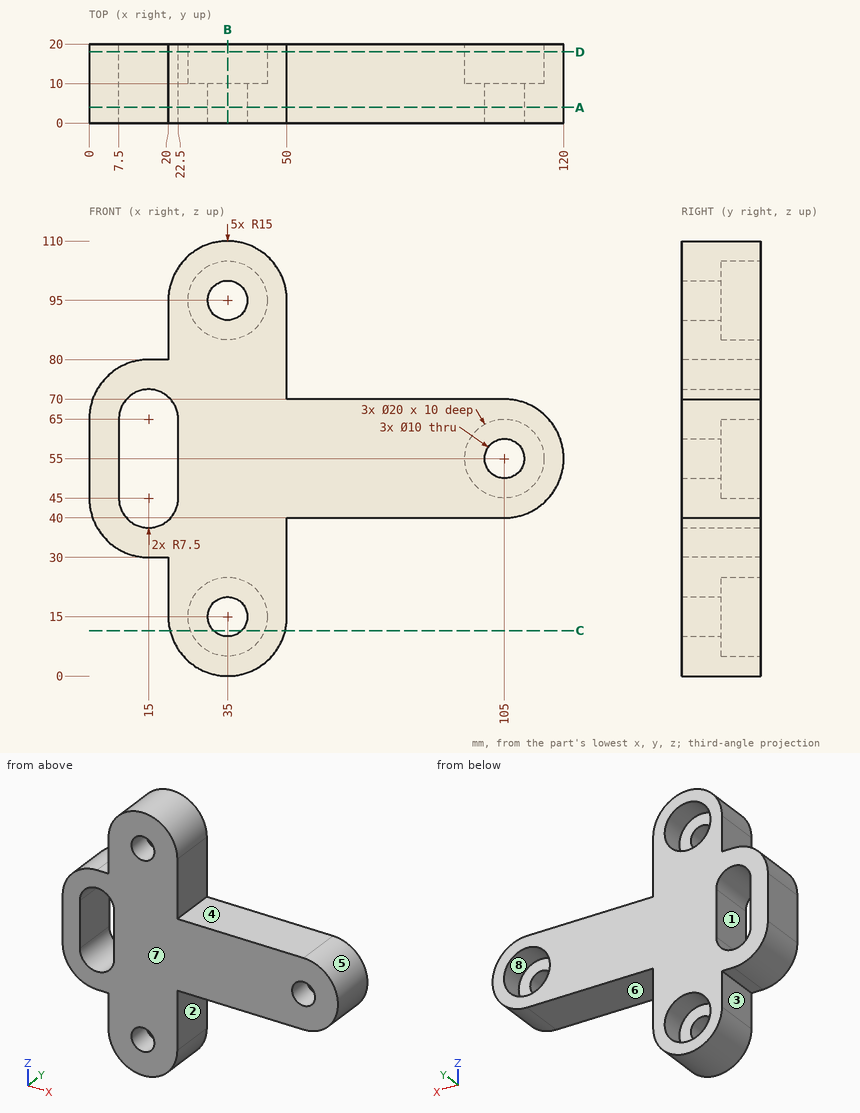
Check sheet for the drawn part. Datum: minimum x, y, z corner. Units: mm. A direction names the side the tool comes from. Give positions to 0.01 mm unless a question says otherwise; leave off trailing zeros. Order: outer loops, then holes, each group sorted by start corner. A loop starts at its lowest first (then second) coordinate and runs counter-clockwise, first axis right, second up. Notation, with made-up numbers: (-33, -31.75) - (4, -31.75) arc R18 cw to (4, -4.75) - close; hole circle Ø3 at (85.25, 49.5). An arc over 180 degrees is marked (long way). Write item = value, one per line. Start each with the question number.
1) Gauge pin test, flat ends, axial feed: pin 1 Ø4 at (y, z) = (10, 64) entering from -X; pin 2 Ø5 at (y, z) = (2.5, 40.5) entering from +X; pin 3 Ø10 at (x, z) = (103, 56.5) entering from +Y; pin 4 Ø1 at (y, z) = (10, 84.5) entering from -X. Record the tip position at first contact, or that the pin passes through.
2) Section check C-C (z = 11.5). Enter the section's corners in (x, y).
3) Section check B-B (x = 35). Enter the section's corners in (y, z).
4) Section check D-D (y = 18). Enter the section's corners in (x, z).
5) Draft check along Z on the marked faces 5, 6, 7 and 8. Enter one of: released by +Z, released by -Z, zero draft, split by the parting line, or undercut.
6) Section check A-A (y = 4). Enter the section's corners in (x, z).
7) Scan lines: L1, parallel to X at y = 6.75, z = 55; L2, parallel to Z at x = 35, y = 14.5; L3, parallel to X at y = 12.75, z = 55. Record each from-to range of solid material in increasing order.
8) Access from +Z, -Z, +X, -X, +Y, -Y to the whole of each face (thin tool, end or side, straight path). Record for the marked faces 1, 2, 3 and 4.
Geometry check:
q1.pin_1 = 0
q1.pin_2 = 114
q1.pin_3 = 10
q1.pin_4 = 20
q2.outline = (20.41, 0) - (31.43, 0) - (31.43, 10) - (25.63, 10) - (25.63, 20) - (20.41, 20) - close; (38.57, 0) - (49.59, 0) - (49.59, 20) - (44.37, 20) - (44.37, 10) - (38.57, 10) - close
q3.outline = (0, 0) - (20, 0) - (20, 5) - (10, 5) - (10, 10) - (0, 10) - close; (0, 20) - (10, 20) - (10, 25) - (20, 25) - (20, 85) - (10, 85) - (10, 90) - (0, 90) - close; (0, 100) - (10, 100) - (10, 105) - (20, 105) - (20, 110) - (0, 110) - close
q4.outline = (0, 45) arc R15 ccw to (15, 30) - (20, 30) - (20, 15) arc R15 ccw to (50, 15) - (50, 40) - (105, 40) arc R15 ccw to (105, 70) - (50, 70) - (50, 95) arc R15 ccw to (20, 95) - (20, 80) - (15, 80) arc R15 ccw to (0, 65) - close; hole (7.5, 45) arc R7.5 ccw to (22.5, 45) - (22.5, 65) arc R7.5 ccw to (7.5, 65) - close; hole circle Ø20 at (35, 15); hole circle Ø20 at (35, 95); hole circle Ø20 at (105, 55)
q5.face_5 = split by the parting line
q5.face_6 = released by -Z
q5.face_7 = zero draft
q5.face_8 = undercut
q6.outline = (0, 45) arc R15 ccw to (15, 30) - (20, 30) - (20, 15) arc R15 ccw to (50, 15) - (50, 40) - (105, 40) arc R15 ccw to (105, 70) - (50, 70) - (50, 95) arc R15 ccw to (20, 95) - (20, 80) - (15, 80) arc R15 ccw to (0, 65) - close; hole (7.5, 45) arc R7.5 ccw to (22.5, 45) - (22.5, 65) arc R7.5 ccw to (7.5, 65) - close; hole circle Ø10 at (35, 15); hole circle Ø10 at (35, 95); hole circle Ø10 at (105, 55)
q7.L1 = 0 to 7.5, 22.5 to 100, 110 to 120
q7.L2 = 0 to 5, 25 to 85, 105 to 110
q7.L3 = 0 to 7.5, 22.5 to 95, 115 to 120
q8.face_1 = +Y, -Y
q8.face_2 = -Z, +X, +Y, -Y
q8.face_3 = -Z, -X, +Y, -Y
q8.face_4 = +Z, +X, +Y, -Y
